```python
from build123d import *

# Parameters (mm, degrees)
SKETCH1_W           = 88.9
SKETCH1_H           = 19.05
BOSS_EXTRUDE1_DEPTH = 19.05
SKETCH2_W           = 6.35
SKETCH2_H           = 19.05
BOSS_EXTRUDE2_DEPTH = 12.7
SKETCH3_R           = 4.445
CUT_EXTRUDE1_DEPTH  = 96.266
SKETCH4_R           = 2.54
CUT_EXTRUDE2_DEPTH  = 96.266
SKETCH5_W           = 53.34
SKETCH5_H           = 19.05
BOSS_EXTRUDE3_DEPTH = 50.8
SKETCH6_W           = 6.35
SKETCH6_H           = 16.51
BOSS_EXTRUDE4_DEPTH = 12.7
SKETCH7_R           = 2.54
CUT_EXTRUDE3_DEPTH  = 61.976
SKETCH8_W           = 19.05
SKETCH8_H           = 10.16
BOSS_EXTRUDE5_DEPTH = 2.54
SKETCH9_W           = 19.05
SKETCH9_H           = 2.54
BOSS_EXTRUDE6_DEPTH = 7.62
SKETCH10_W          = 38.1
SKETCH10_H          = 19.05
BOSS_EXTRUDE7_DEPTH = 25.4
SKETCH11_R          = 6.35
CUT_EXTRUDE4_DEPTH  = 12.7


with BuildPart() as part:
    # Sketch1 → Boss-Extrude1 (new body)
    with BuildSketch(Plane.XY):
        with Locations((44.45, -9.525)):
            Rectangle(SKETCH1_W, SKETCH1_H)
    extrude(amount=BOSS_EXTRUDE1_DEPTH)

    # Sketch2 → Boss-Extrude2 (add)
    with BuildSketch(Plane.XZ.offset(19.05)):
        with Locations((21.758870797, 9.525)):
            Rectangle(SKETCH2_W, SKETCH2_H)
        with Locations((68.748870797, 9.525)):
            Rectangle(SKETCH2_W, SKETCH2_H)
    extrude(amount=BOSS_EXTRUDE2_DEPTH)

    # Sketch3 → Cut-Extrude1 (cut)
    with BuildSketch(Plane.ZY):
        with Locations((9.525, -9.525)):
            Circle(SKETCH3_R)
    extrude(amount=-CUT_EXTRUDE1_DEPTH, mode=Mode.SUBTRACT)

    # Sketch4 → Cut-Extrude2 (cut)
    with BuildSketch(Plane.ZY.offset(-18.583870797)):
        with Locations((9.525, -25.4)):
            Circle(SKETCH4_R)
    extrude(amount=-CUT_EXTRUDE2_DEPTH, mode=Mode.SUBTRACT)

    # Sketch5 → Boss-Extrude3 (add)
    with BuildSketch(Plane.XY.offset(19.05)):
        with Locations((45.253870797, -9.525)):
            Rectangle(SKETCH5_W, SKETCH5_H)
    extrude(amount=BOSS_EXTRUDE3_DEPTH)

    # Sketch6 → Boss-Extrude4 (add)
    with BuildSketch(Plane.XZ.offset(19.05)):
        with Locations((21.758870797, 61.595)):
            Rectangle(SKETCH6_W, SKETCH6_H)
        with Locations((68.748870797, 61.595)):
            Rectangle(SKETCH6_W, SKETCH6_H)
    extrude(amount=BOSS_EXTRUDE4_DEPTH)

    # Sketch7 → Cut-Extrude3 (cut)
    with BuildSketch(Plane.ZY.offset(-18.583870797)):
        with Locations((61.595, -26.67)):
            Circle(SKETCH7_R)
    extrude(amount=-CUT_EXTRUDE3_DEPTH, mode=Mode.SUBTRACT)

    # Sketch8 → Boss-Extrude5 (add)
    with BuildSketch(Plane(origin=(0, 0, 0), x_dir=(1, 0, 0), z_dir=(0, 1, 0))):
        with Locations((44.45, -5.08)):
            Rectangle(SKETCH8_W, SKETCH8_H)
    extrude(amount=BOSS_EXTRUDE5_DEPTH)

    # Sketch9 → Boss-Extrude6 (add)
    with BuildSketch(Plane(origin=(0, 2.54, 0), x_dir=(1, 0, 0), z_dir=(0, 1, 0))):
        with Locations((44.45, -1.27)):
            Rectangle(SKETCH9_W, SKETCH9_H)
        with Locations((44.45, -8.89)):
            Rectangle(SKETCH9_W, SKETCH9_H)
    extrude(amount=BOSS_EXTRUDE6_DEPTH)

    # Sketch10 → Boss-Extrude7 (add)
    with BuildSketch(Plane.XY.offset(69.85)):
        with Locations((45.253870797, -9.525)):
            Rectangle(SKETCH10_W, SKETCH10_H)
    extrude(amount=BOSS_EXTRUDE7_DEPTH)

    # Sketch11 → Cut-Extrude4 (cut)
    with BuildSketch(Plane.ZY.offset(-26.203870797)):
        with Locations((82.55, -9.525)):
            Circle(SKETCH11_R)
    extrude(amount=-CUT_EXTRUDE4_DEPTH, mode=Mode.SUBTRACT)


solid = part.part
```
Design review of the part built by this model. Coordinates are the model's own, in mm. A direction names the side the tool comes from. Coordinates: 2 decimals unless noted, no trailing zeros. Order: outer loops, then holes, each group sorted by start corner. A loop starts at its lowest first (then second) coordinate and runs counter-clockwise, first axis right, second up. Notation, with made-up numbers: (-37.5, 47) - (-11.5, 47) arc R10 cw to (-11.5, 60) - close; hole circle Ø11 at (-36.75, 20). An arc over 180 degrees is marked (long way). One line per question, with ' | ' between items.
Q1. Consider section C-C, the plane y = -25.4. Give the number of separate pieces and of enclosed holes in the cut face, then the cut area to 3 significant figures.
Answer key:
separate pieces: 8 | enclosed holes: 0 | area: 331 mm2
Q2. For faces 1 (the flat face through (53.975, 2, 5)), 2 (the flat face through (65.574, -24, 61)), 3 (the flat face through (18.584, -24, 7)), 4 (the flat face through (22, -25, 19.05)), 5 (the flat face through (26.204, -16, 85)), list the 3-axis set-ups (+Z, -Z, +X, -X, +Y, -Y) from which the entire face can be reached by the end or side of a thin tool; tool diameter is ignored.
Answer key:
face 1: +Z, -Z, +X, +Y | face 2: +Z, -Z, -Y | face 3: +Z, -Z, -X, -Y | face 4: +X, -X, -Y | face 5: +Z, -X, +Y, -Y
Q3. Consider section D-D, the plane x = 9.5. Give the boundary of the cut face in (y, z) (3 decimals).
Answer key:
outline: (-19.05, 0) - (0, 0) - (0, 19.05) - (-19.05, 19.05) - close; hole circle Ø8.89 at (-9.525, 9.525)
Q4. Consider section A-A, the plane y = 4.5. Give the boundary of the cut face in (x, z) (3 decimals), then the cut area to 3 significant figures.
Answer key:
outline: (34.925, 0) - (53.975, 0) - (53.975, 2.54) - (34.925, 2.54) - close; (34.925, 7.62) - (53.975, 7.62) - (53.975, 10.16) - (34.925, 10.16) - close | area: 96.8 mm2
Q5. Clearance check with flat-ended pins moving along their axes: pin 1 Ø10 at (y, z) = (-27.5, 8.5) entering from +X; pin 2 Ø6 at (x, y) = (21.5, -7) entering from -Z; pin 3 Ø15 at (x, z) = (8, 11) entering from -Y; pin 4 Ø3 at (x, y) = (70, -24) entering from +Z. State where each tip first meets the part, or that it passes through.
Answer key:
pin 1: stops at x = 71.92 | pin 2: stops at z = 0 | pin 3: stops at y = -19.05 | pin 4: stops at z = 69.85
Q6. Consider section B-B, the plane z = 82.55. Give the boundary of the cut face in (x, y) (3 decimals), then the cut area to 3 significant figures.
Answer key:
outline: (26.204, -19.05) - (64.304, -19.05) - (64.304, 0) - (26.204, 0) - (26.204, -3.175) - (38.904, -3.175) - (38.904, -15.875) - (26.204, -15.875) - close | area: 565 mm2
Q7. The part is to be moulded in two halves that separate along Y. For faces 6 (the flat face through (69, -25, 19.05)), 7 (the cylindrical face through (43.828, -13.468, 11.576)), 8 (the flat face through (22, -31.75, 10)), 9 (the flat face through (44, 10.16, 1)), say which applies: +Y half, -Y half, draft (parallel to the pull), parting line (faces both ways), or undercut.
Answer key:
face 6: draft | face 7: undercut | face 8: -Y half | face 9: +Y half
Q8. To check wall thickness, follow line 1 along X through (y, z) = (-25, 64.5); line 2 along Z through (x, y) = (70, -24.5); line 3 along Y through (x, z) = (56, 26.5). State the ranges of each line that lie inside material, in increasing order.
Answer key:
line 1: x = 18.58 to 24.93, 65.57 to 71.92 | line 2: z = 0 to 7.15, 11.9 to 19.05, 53.34 to 60.27, 62.92 to 69.85 | line 3: y = -19.05 to 0
